Geometry: see drawing. Coordinates: mm, zero at the bounding-box minimum. A direction names the side the tool comes from. Round coordinates to 2 decimals unless told otherwise and drop trailing zeros. Loops run counter-clockwise (first coordinate to the right, second up) from the corner with the lowest first, then second, coordinate; pieces in that order, holes last.
(1) Material intervals for probe 1 along Y at (x, z) = (122, 36.5); probe 2 along Y at (x, z) = (94.5, 37); probe 3 along Z at (x, y) = (124.5, 109), sorted ascending.
(2) Section C-C, the plane y = 61. Return the cut outline in (x, z), plus the area to 3 significant figures.
(3) Section A-A, the plane x = 33.5. Return the cut outline in (y, z), plus the area to 3 significant figures.
(4) First-contact query: pin 1 Ø10 at (x, z) = (48.5, 35.5) entering from -Y. Flat tip, straight axial feed; report the tip coordinate or a pass-through.
(5) Set-up query: the marked faces 1 and 2. Return all of +Z, -Z, +X, -X, +Y, -Y with unobstructed straight access to the full face (end or side cutting, diameter ignored); none if empty.
(6) Section B-B, the plane z = 38.5. Return the cut outline in (x, y).
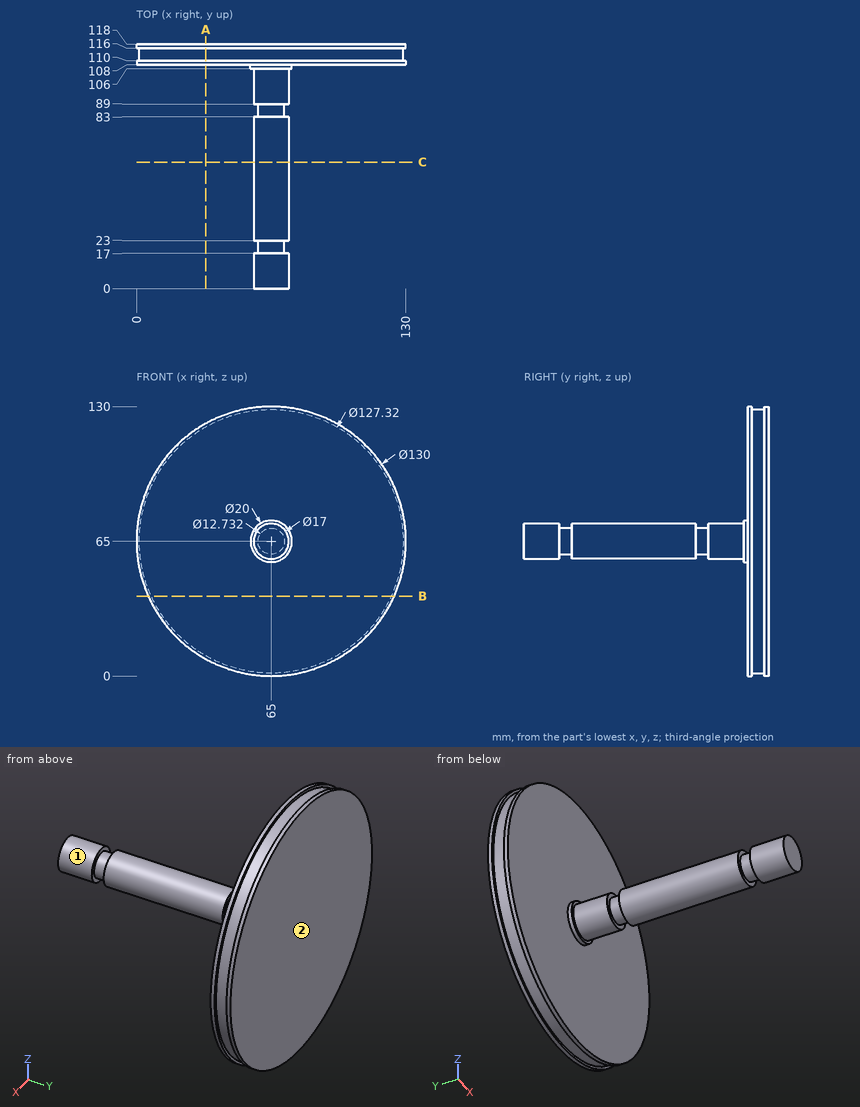
Output values:
1. probe 1: y = 108 to 110, 116 to 118
1. probe 2: y = 108 to 118
1. probe 3: z = 38.83 to 91.17
2. outline: circle Ø17 at (65, 65)
2. area: 227 mm2
3. outline: (108, 8.14) - (110, 8.14) - (110, 9.68) - (116, 9.68) - (116, 8.14) - (118, 8.14) - (118, 121.86) - (116, 121.86) - (116, 120.32) - (110, 120.32) - (110, 121.86) - (108, 121.86) - close
3. area: 1,120 mm2
4. pin 1: stops at y = 108
5. face 1: -Y
5. face 2: +Z, -Z, +X, -X, +Y
6. outline: (5.65, 108) - (124.35, 108) - (124.35, 110) - (122.88, 110) - (122.88, 116) - (124.35, 116) - (124.35, 118) - (5.65, 118) - (5.65, 116) - (7.12, 116) - (7.12, 110) - (5.65, 110) - close
